Could you check a few things on this model? Use its own coordinates, in mm. Face numbers are marked on the shaded views. A direction names the side the tool comes from. Round coordinates to 2 decimals unless told otherwise and drop trailing zeros. Order: outer loops, then holes, each group sorted by start corner. A loop starts at its lowest first (then second) coordinate and runs counter-clockwise, first axis right, second up. Notation, with made-up numbers: M -27.5,75 L 9.5,75 A20 ccw 9.5,113 Z; hole C 16.5,42 d1. An arc over 180 degrees is marked long. Write each question's results on one line, items separated by ' | '. Start each with the question number.
1. I'm going to push flat-ended pins straight in: pin 1 (14.5 mm diameter, centred on x = 5.5, z = 41, fed in from +Y); pin 2 (8.5 mm diameter, centred on y = 1, z = 48.5, fed in from -X); pin 3 (3 mm diameter, centred on x = 7, z = 11.5, fed in from -Y). Where does each tip first touch, or does it pass through?
2. Suppose I cut it at C-C on y = 16.5. Write out the boundary of the cut face in (x, z), and give its area (3 significant figures).
3. We'd pull the mould along Z, two halves only. Please class the marked faces 5, 6, 7 and 8: released by +Z, released by -Z, zero draft, split by the parting line, or undercut.
4. Suppose I cut it at D-D on x = 0. Write out the boundary of the cut face in (y, z).
5. Suppose I cut it at A-A on y = 0. Write out the boundary of the cut face in (x, z).
6. Suppose I cut it at B-B on x = 14.5. Write out the boundary of the cut face in (y, z), and give its area (3 significant figures).
7. Please list where these lines run through material, in increasing order: L1, parallel to Z at x = -19, y = 15.5; L2, parallel to Z at x = 24, y = 12.5; L3, parallel to X at y = 15, z = 45.
8. For the marked faces 1, 2, 3 and 4, which set-ups out of +Z, -Z, +X, -X, +Y, -Y let a thin tool reach every point of the face, with its end or its side?
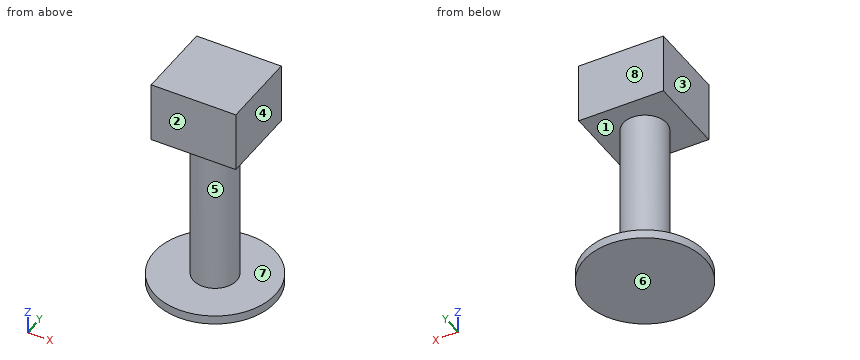
from build123d import *

# Parameters (mm, degrees)
F0_W     = 10.3772366419
F0_H     = 78.2052613795
F3_START = 32.766
F2_W     = 40.606578812
F2_H     = 37.899473682
F3_DEPTH = 28.956


with BuildPart() as f1:
    # F0 (on Front) → F1 (revolve)
    with BuildSketch(Plane.XZ):
        with Locations((-5.188618321, -3.4590791911)):
            Rectangle(F0_W, F0_H)
        Polygon((-29.026184231, -46.772763133), (0, -46.772763133), (0, -42.5617098808), (-10.3772366419, -42.5617098808), (-29.026184231, -42.5617098808), align=None)
    revolve(axis=Axis((0, 0, -3.4590791911), (0, 0, -1)))

    # F2 (on Top) → F3 (join)
    with BuildSketch(Plane.XY.offset(F3_START)):
        with Locations((0.3007883206, 0.4511838779)):
            Rectangle(F2_W, F2_H)
    extrude(amount=F3_DEPTH)


solid = f1.part
Filled sheet:
1) pin 1: stops at y = 19.4 | pin 2: stops at x = -20 | pin 3: stops at y = -8.8
2) outline: M -23.88,-46.77 L 23.88,-46.77 L 23.88,-42.56 L -23.88,-42.56 Z; M -20,32.77 L 20.6,32.77 L 20.6,61.72 L -20,61.72 Z | area: 1,380 mm^2
3) face 5: undercut | face 6: released by -Z | face 7: undercut | face 8: zero draft
4) outline: M -29.03,-46.77 L 29.03,-46.77 L 29.03,-42.56 L 10.38,-42.56 L 10.38,32.77 L 19.4,32.77 L 19.4,61.72 L -18.5,61.72 L -18.5,32.77 L -10.38,32.77 L -10.38,-42.56 L -29.03,-42.56 Z
5) outline: M -29.03,-46.77 L 29.03,-46.77 L 29.03,-42.56 L 10.38,-42.56 L 10.38,32.77 L 20.6,32.77 L 20.6,61.72 L -20,61.72 L -20,32.77 L -10.38,32.77 L -10.38,-42.56 L -29.03,-42.56 Z
6) outline: M -25.14,-46.77 L 25.14,-46.77 L 25.14,-42.56 L -25.14,-42.56 Z; M -18.5,32.77 L 19.4,32.77 L 19.4,61.72 L -18.5,61.72 Z | area: 1,310 mm^2
7) L1: z = -46.77 to -42.56, 32.77 to 61.72 | L2: z = -46.77 to -42.56 | L3: x = -20 to 20.6
8) face 1: none | face 2: +Z, +X, -X, -Y | face 3: +Z, -X, +Y, -Y | face 4: +Z, +X, +Y, -Y
